Verification items for this drawing (mm, ordinates from the low corner). A direction names the side the tool comes from. Give positions to 0.01 mm unless a question says otherwise; leave off trailing zeros. Loops run counter-clockwise (first coordinate to the right, second up) from the corner with the lowest first, then second, coordinate; pieces in that order, holes last. Notation, with made-up numbers: M 77.25,12 L 115.25,12 A10 cw 115.25,27 Z; hole C 55,-33 d9. An arc over 180 degrees is marked long. Use a Markdown table: item, result.
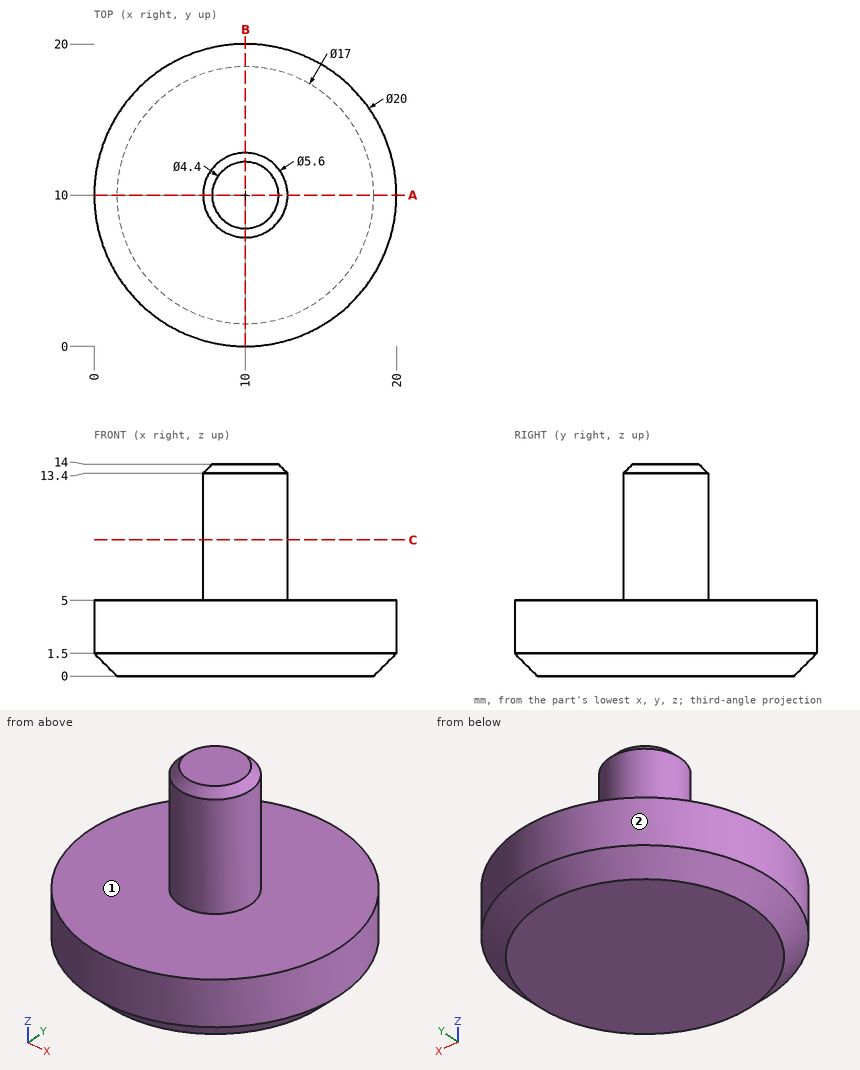
(1) Material ranges on line 1 (Z direction, x = 12.5, y = 12); line 2 (Y direction, x = 10, z = 6); line 3 (X direction, y = 7.5, z = 8.5), recorded low to high.
Results below:
| item | result |
|---|---|
| line 1 | 0 to 5 |
| line 2 | 7.2 to 12.8 |
| line 3 | 8.74 to 11.26 |
(2) Set-up check for the marked faces 1 and 2: record each of +Z, -Z, +X, -X, +Y, -Y from which the full face is reachable in a straight line by a thin tool's end or side.
Results below:
| item | result |
|---|---|
| face 1 | +Z |
| face 2 | +Z, -Z |
(3) Gauge pin test, flat ends, axial feed: P1, Ø5, axis at x = 14, z = 3, coming from the -Y side; P2, Ø1.5, axis at x = 16.5, y = 7, coming from the -Z side; P3, Ø1, axis at x = 14.5, y = 14.5, coming from the +Z side; P4, Ø3, axis at y = 12.5, z = 6, coming from the +X side. Record the tip position at first contact, or that the pin passes through.
Results below:
| item | result |
|---|---|
| P1 | y = 0.11 |
| P2 | z = 0 |
| P3 | z = 5 |
| P4 | x = 19.9 |
(4) Cross-section at C-C on z = 9. Record the cut outline in (x, y).
Results below:
| item | result |
|---|---|
| outline | C 10,10 d5.6 |
(5) Cross-section at A-A on y = 10. Record the cut outline in (x, z).
Results below:
| item | result |
|---|---|
| outline | M 0,1.5 L 1.5,0 L 18.5,0 L 20,1.5 L 20,5 L 12.8,5 L 12.8,13.4 L 12.2,14 L 7.8,14 L 7.2,13.4 L 7.2,5 L 0,5 Z |
